```python
from build123d import *

# Parameters (mm, degrees)
TABAN_FLAN_1_DEPTH    = 400
IZIM2_R               = 4.25
KES_EKSTR_ZYON1_DEPTH = 10
IZIM3_R               = 3.25
KES_EKSTR_ZYON2_DEPTH = 10


# Sheet-metal steps are written as plain solids
with BuildPart() as part:
    # Çizim1 → Taban-Flanş1 (new, symmetric)
    with BuildSketch(Plane.XY):
        with BuildLine():
            Line((-195, 400), (-195, 2.2366))
            ThreePointArc((-195, 2.2366), (-194.344915027, 0.655084973), (-192.7634, 0))
            Line((-192.7634, 0), (192.7634, 0))
            ThreePointArc((192.7634, 0), (194.344915027, 0.655084973), (195, 2.2366))
            Line((195, 2.2366), (195, 400))
            Line((195, 400), (193.5, 400))
            Line((193.5, 400), (193.5, 2.2366))
            ThreePointArc((193.5, 2.2366), (193.284254855, 1.715745145), (192.7634, 1.5))
            Line((192.7634, 1.5), (-192.7634, 1.5))
            ThreePointArc((-192.7634, 1.5), (-193.284254855, 1.715745145), (-193.5, 2.2366))
            Line((-193.5, 2.2366), (-193.5, 400))
            Line((-193.5, 400), (-195, 400))
        make_face()
    extrude(amount=TABAN_FLAN_1_DEPTH, both=True)

    # Çizim2 → Kes-Ekstrüzyon1 (cut)
    with BuildSketch(Plane(origin=(-193.5, 0, 0), x_dir=(0, 0, -1), z_dir=(1, 0, 0))):
        with Locations((307.5, 350.5)):
            Circle(IZIM2_R)
        with Locations((307.5, 236.5)):
            Circle(IZIM2_R)
        with Locations(Location((-307.5, 236.5, 0), (0, 0, 180))):
            Circle(IZIM2_R)
        with Locations(Location((-307.5, 350.5, 0), (0, 0, 180))):
            Circle(IZIM2_R)
    extrude(amount=-KES_EKSTR_ZYON1_DEPTH, mode=Mode.SUBTRACT)

    # Çizim3 → Kes-Ekstrüzyon2 (cut)
    with BuildSketch(Plane.XZ):
        with Locations((-175, 338.5)):
            Circle(IZIM3_R)
        with Locations((-129, 338.5)):
            Circle(IZIM3_R)
        with Locations((175, 338.5)):
            Circle(IZIM3_R)
        with Locations((129, 338.5)):
            Circle(IZIM3_R)
        with Locations((-175, -338.5)):
            Circle(IZIM3_R)
        with Locations((-129, -338.5)):
            Circle(IZIM3_R)
        with Locations((129, -338.5)):
            Circle(IZIM3_R)
        with Locations((175, -338.5)):
            Circle(IZIM3_R)
    extrude(amount=-KES_EKSTR_ZYON2_DEPTH, mode=Mode.SUBTRACT)


solid = part.part
```
Work out the finished part from the listing and answer in its coordinate system (mm). A direction names the side the tool comes from. Give positions to 0.01 mm unless a question says otherwise; leave off trailing zeros. Loops run counter-clockwise (first coordinate to the right, second up) from the corner with the lowest first, then second, coordinate; pieces in that order, holes last. Notation, with made-up numbers: (50.5, -30.75) -> (107.5, -30.75) arc R26 cw to (107.5, 4.25) -> close; hole circle Ø6 at (50.5, 37). An arc over 180 degrees is marked (long way). Use CSV: the item, a comma, the result in double quotes.
1. The part is cut by section A-A (y = 26.5). Write down the section's boundary in (x, z), then the cut area to 3 significant figures.
Found:
outline,"(-195, -400) -> (-193.5, -400) -> (-193.5, 400) -> (-195, 400) -> close; (193.5, -400) -> (195, -400) -> (195, 400) -> (193.5, 400) -> close"
area,"2,400 mm^2"
2. A tool of negligible diameter and unlimited length cuts with its end or side. For faces 4 (the flat face through (-195, 204, 6)), 5 (the flat face through (3, 1.5, 6)), from which of +Z, -Z, +X, -X, +Y, -Y can it reach the whole face along a straight path? Write none if from no direction.
Found:
face 4,"+Z, -Z, -X, +Y, -Y"
face 5,"+Z, -Z, +Y"
3. The part is cut by section B-B (z = 272). Write down the section's boundary in (x, y), then the cut area to 3 significant figures.
Found:
outline,"(-195, 2.24) arc R2.24 ccw to (-192.76, 0) -> (192.76, 0) arc R2.24 ccw to (195, 2.24) -> (195, 400) -> (193.5, 400) -> (193.5, 2.24) arc R0.74 cw to (192.76, 1.5) -> (-192.76, 1.5) arc R0.74 cw to (-193.5, 2.24) -> (-193.5, 400) -> (-195, 400) -> close"
area,"1,780 mm^2"
4. The part is cut by section C-C (x = 117). Write down the section's boundary in (y, z).
Found:
outline,"(0, -400) -> (1.5, -400) -> (1.5, 400) -> (0, 400) -> close"
5. Flat-ended cylindrical pins translate along their axes: pin 1 Ø7.5 at (x, z) = (129, 338.5) entering from +Y; pin 2 Ø5 at (x, z) = (175, 338.5) entering from +Y. Find the tip coordinate at first contact, or state that the pin passes through.
Found:
pin 1,"y = 1.5"
pin 2,"through"
6. Straight lines are drawn through the part: line 1 (X direction, y = 197, z = 129); line 2 (Z direction, x = -194.5, y = 350.5); line 3 (Y direction, x = -193.9, z = -307.5). For each, find the intervals that lie inside material, in ascending order.
Found:
line 1,"-195 to -193.5, 193.5 to 195"
line 2,"-400 to -311.75, -303.25 to 303.25, 311.75 to 400"
line 3,"0.31 to 232.25, 240.75 to 346.25, 354.75 to 400"
7. The mould has two halves that part along X. Classify faces 1 (the flat face through (195, 198, 6)), 2 (the flat face through (-3, 0, 6)), 3 (the flat face through (193.5, 204, 6)): +X half, -X half, draft (parallel to the pull), parting line (faces both ways), or undercut.
Found:
face 1,"+X half"
face 2,"draft"
face 3,"undercut"
